```python
from build123d import *

# Parameters (mm, degrees)
BOSS_EXTRUDE1_DEPTH = 24
SKETCH5_R           = 6.5
BOSS_EXTRUDE3_DEPTH = 29.899298
SKETCH3_R           = 3
CUT_EXTRUDE1_DEPTH  = 30.899298428
FILLET1_R           = 3
CHAMFER1_SIZE       = 1


with BuildPart() as part:
    # Sketch1 → Boss-Extrude1 (new body)
    with BuildSketch(Plane.XY):
        Polygon((0, 15), (14.899298428, 15), (14.899298428, -14.949649214), (-15, -14.949649214), (-15, 15), align=None)
        Polygon((-9.966432809, 9.966432809), (-4.741432809, 9.966432809), (-3.1, 8.307461143), (-5.5, 8.307461143), (-5.5, 6.667461143), (-2.79, 3.957461143), (2.79, 3.957461143), (5.5, 6.667461143), (5.5, 8.307461143), (3.1, 8.307461143), (4.741432809, 9.966432809), (9.966432809, 9.966432809), (9.966432809, 4.741432809), (8.307461143, 3.1), (8.307461143, 5.5), (6.667461143, 5.5), (3.957461143, 2.79), (3.957461143, -2.79), (6.667461143, -5.5), (8.307461143, -5.5), (8.307461143, -3.1), (9.966432809, -4.741432809), (9.966432809, -9.966432809), (4.741432809, -9.966432809), (3.1, -8.307461143), (5.5, -8.307461143), (5.5, -6.667461143), (2.79, -3.957461143), (-2.79, -3.957461143), (-5.5, -6.667461143), (-5.5, -8.307461143), (-3.1, -8.307461143), (-4.741432809, -9.966432809), (-9.966432809, -9.966432809), (-9.966432809, -4.741432809), (-8.307461143, -3.1), (-8.307461143, -5.5), (-6.667461143, -5.5), (-3.957461143, -2.79), (-3.957461143, 2.79), (-6.667461143, 5.5), (-8.307461143, 5.5), (-8.307461143, 3.1), (-9.966432809, 4.741432809), align=None, mode=Mode.SUBTRACT)
    extrude(amount=BOSS_EXTRUDE1_DEPTH)

    # Sketch5 → Boss-Extrude3 (add, through all)
    with BuildSketch(Plane.ZY.offset(15)):
        with BuildLine():
            Line((0, 15), (24, 15))
            Line((24, 15), (24, 23.5))
            ThreePointArc((24, 23.5), (12, 35.5), (0, 23.5))
            Line((0, 23.5), (0, 15))
        make_face()
        with Locations((12, 23.5)):
            Circle(SKETCH5_R, mode=Mode.SUBTRACT)
    extrude(amount=-BOSS_EXTRUDE3_DEPTH)

    # Sketch3 → Cut-Extrude1 (cut, through all)
    with BuildSketch(Plane.ZY.offset(15)):
        with Locations((12, 0)):
            Circle(SKETCH3_R)
    extrude(amount=-CUT_EXTRUDE1_DEPTH, mode=Mode.SUBTRACT)

    # Fillet1
    fillet1_edges = [part.edges().sort_by_distance(p)[0] for p in [
        (-0.050350786, -14.949649214, 24),
        (14.899298428, 0.025175393, 24),
        (14.899298, 35.5, 12),
        (-15, 35.5, 12),
        (14.899298428, 0.025175393, 0),
        (-0.050350786, -14.949649214, 0),
        (-15, 4.275175393, 0),
        (-15, 4.275175393, 24),
        (14.899298428, -14.949649214, 12),
        (-15, -14.949649214, 12),
    ]]
    fillet(fillet1_edges, radius=FILLET1_R)

    # Chamfer1
    chamfer1_edges = [part.edges().sort_by_distance(p)[0] for p in [
        (14.899298, 23.5, 5.5),
        (-15, 23.5, 5.5),
        (14.899298428, 0, 9),
        (-15, 0, 9),
    ]]
    chamfer(chamfer1_edges, length=CHAMFER1_SIZE)


solid = part.part
```
Can you work these out from the model? Positions are in its coordinate system, mm. Round coordinates to 2 decimals unless told otherwise and drop trailing zeros. Loops run counter-clockwise (first coordinate to the right, second up) from the corner with the lowest first, then second, coordinate; pieces in that order, holes last. Notation, with made-up numbers: M -0.5,-1 L 57.5,-1 A7 ccw 57.5,4 Z; hole C 71,-33 d2. An arc over 180 degrees is marked long. Answer in a Markdown table with one row per item.
1. Please list where these lines run through material, in increasing order: line 1 (Y direction, x = 2, z = 12); line 2 (Y direction, x = -8, z = 12); line 3 (X direction, y = 8, z = 11.25). Write a range as from..to.
Established:
| item | result |
|---|---|
| line 1 | -14.95..-3.96, 3.96..17, 30..35.5 |
| line 2 | -14.95..-9.97, -5.5..-3, 3..5.5, 9.97..17, 30..35.5 |
| line 3 | -15..-9.97, -5.5..5.5, 9.97..14.9 |
2. If we section it at B-B, the plane z = 17.5: Give the number of separate pieces and of enclosed holes in the cut face, plus the area to 3 significant figures.
Established:
| item | result |
|---|---|
| separate pieces | 2 |
| enclosed holes | 1 |
| area | 1,070 mm² |
3. If we section it at A-A, the plane y = 0: Please give me the cut outline in (x, z).
Established:
| item | result |
|---|---|
| outline | M -15,3 A3 ccw -12,0 L -3.96,0 L -3.96,9 L -14,9 L -15,8 Z; M -15,16 L -14,15 L -3.96,15 L -3.96,24 L -12,24 A3 ccw -15,21 Z; M 3.96,0 L 11.9,0 A3 ccw 14.9,3 L 14.9,8 L 13.9,9 L 3.96,9 Z; M 3.96,15 L 13.9,15 L 14.9,16 L 14.9,21 A3 ccw 11.9,24 L 3.96,24 Z |
4. I'm going to push flat-ended pins straight in: pin 1 Ø1.3 at (x, z) = (7, 17.5) entering from +Y; pin 2 Ø1.9 at (x, z) = (-4.5, 9) entering from +Y; pin 3 Ø1.5 at (x, z) = (10.5, 8.5) entering from +Y. Where does each tip first touch, or does it pass through?
Established:
| item | result |
|---|---|
| pin 1 | y = 34.48 |
| pin 2 | y = 35.32 |
| pin 3 | y = 35.18 |
